Read the model definition and answer for the solid it produces. Units are mm, in the model's axes. A direction names the side the tool comes from. Give positions to 0.01 mm unless a question says otherwise; leave off trailing zeros. Write each loop counter-clockwise with the first axis right and the second up, starting at its lowest first coordinate (ties: lowest second). Pieces come first, ordered by that corner, then holes. Notation, with made-up numbers: (33.25, 69) - (43.25, 69) arc R21 cw to (43.25, 102) - close; hole circle Ø6 at (47.25, 89). An arc over 180 degrees is marked (long way). Answer as CSV lines item,"result".
```python
from build123d import *

# Parameters (mm, degrees)
TUBE_R                   = 5
TUBE_R_2                 = 4
TUBE_DEPTH               = 24
TUBE_PLACEMENT_ANGLE     = 70
BOX002_W                 = 13
BOX002_H                 = 4
BOX002_DEPTH             = 16
BOX001_W                 = 15
BOX001_H                 = 5
BOX001_DEPTH             = 18
CYLINDER_R               = 4
CYLINDER_DEPTH           = 35
CYLINDER_PLACEMENT_ANGLE = 70
BOX_W                    = 50
BOX_H                    = 100
BOX_DEPTH                = 2.6
EXTRUDE_DEPTH            = 10
EXTRUDE_PLACEMENT_ANGLE  = 70


with BuildPart() as tube:
    # Tube → Tube (new body)
    with BuildSketch(Plane.XY):
        Circle(TUBE_R)
        Circle(TUBE_R_2, mode=Mode.SUBTRACT)
    extrude(amount=TUBE_DEPTH)


with BuildPart() as tube_1:
    # Tube placement: moved
    add(tube.part.moved(Location((25.1, 89, -0.7))).rotate(Axis((25.1, 89, -0.7), (1, 0, 0)), TUBE_PLACEMENT_ANGLE))


with BuildPart() as cube002:
    # Box002 → Box002 (new body)
    with BuildSketch(Plane(origin=(18.5, 45, -6), x_dir=(1, 0, 0), z_dir=(0, 0, 1))):
        with Locations((6.5, 2)):
            Rectangle(BOX002_W, BOX002_H)
    extrude(amount=BOX002_DEPTH)


with BuildPart() as cut001:
    # Box001 → Box001 (new body)
    with BuildSketch(Plane(origin=(17.5, 45, -7.13), x_dir=(1, 0, 0), z_dir=(0, 0, 1))):
        with Locations((7.5, 2.5)):
            Rectangle(BOX001_W, BOX001_H)
    extrude(amount=BOX001_DEPTH)

    # Cut001: cut Cube002
    add(cube002.part, mode=Mode.SUBTRACT)


with BuildPart() as cut001_1:
    # Cut001 placement: moved
    add(cut001.part.moved(Location((0, 50, -8.5))))


with BuildPart() as cylinder:
    # Cylinder → Cylinder (new body)
    with BuildSketch(Plane.XY):
        Circle(CYLINDER_R)
    extrude(amount=CYLINDER_DEPTH)


with BuildPart() as cylinder_1:
    # Cylinder placement: moved
    add(cylinder.part.moved(Location((25.1, 98, -4))).rotate(Axis((25.1, 98, -4), (1, 0, 0)), CYLINDER_PLACEMENT_ANGLE))


with BuildPart() as cut:
    # Box → Box (new body)
    with BuildSketch(Plane.XY):
        with Locations((25, 50)):
            Rectangle(BOX_W, BOX_H)
    extrude(amount=BOX_DEPTH)

    # Cut: cut Cylinder
    add(cylinder_1.part, mode=Mode.SUBTRACT)


with BuildPart() as fusion:
    # Sketch → Extrude (new body)
    with BuildSketch(Plane.XY):
        with BuildLine():
            ThreePointArc((29.005047, 25.145956), (25.102383, 29.048619), (21.199722, 25.145954))
            Line((21.199722, 25.145954), (20.095131, 25.124403))
            ThreePointArc((30.109684, 25.145956), (25.091608, 30.153244), (20.095131, 25.124403))
            Line((29.005047, 25.145956), (30.109684, 25.145956))
        make_face()
    extrude(amount=EXTRUDE_DEPTH)


with BuildPart() as fusion_1:
    # Extrude placement: moved
    add(fusion.part.moved(Location((0, 89.5, -27.7))).rotate(Axis((0, 89.5, -27.7), (1, 0, 0)), EXTRUDE_PLACEMENT_ANGLE))

    # Fusion: union Tube, Cut001, Cut
    add(tube_1.part)
    add(cut001_1.part)
    add(cut.part)


solid = fusion_1.part
```
(1) Find the intervals of material crossed by L1, parallel to X at y = 82, z = 1.5; L2, parallel to Z at x = 47, y = 28; L3, parallel to Y at x = 27.5, z = -8.25, in increasing order.
Worked out:
L1,"x = 0 to 21.11, 29.09 to 50"
L2,"z = 0 to 2.6"
L3,"y = 99 to 100"
(2) A cutting plane is placed at C-C (y = 38). Write down the section's boundary in (x, z).
Worked out:
outline,"(0, 0) - (50, 0) - (50, 2.6) - (0, 2.6) - close"
(3) A cutting plane is placed at B-B (x = 39.5). Write down the section's boundary in (y, z), and give its area (3 significant figures).
Worked out:
outline,"(0, 0) - (100, 0) - (100, 2.6) - (0, 2.6) - close"
area,"260 mm^2"
(4) For faces 1 (the flat face through (18.5, 97, -7)), 2 (the flat face through (25, 0, 1)), 3 (the flat face through (32.5, 97, -8)), 4 (the cylindrical face through (20.456, 95.15, -1.012)), determine the directions among +Z, -Z, +X, -X, +Y, -Y from which every point of the face is accessible in a straight line to the end or side of a thin tool.
Worked out:
face 1,"-Y"
face 2,"+Z, -Z, +X, -X, -Y"
face 3,"-Z, +X, +Y, -Y"
face 4,"none"
(5) A cutting plane is placed at A-A (z = -6.75). Write down the section's boundary in (x, y), and give its area (3 significant figures).
Worked out:
outline,"(17.5, 95) - (18.5, 95) - (18.5, 99) - (31.5, 99) - (31.5, 95) - (32.5, 95) - (32.5, 100) - (17.5, 100) - close"
area,"23.0 mm^2"
(6) Each of these flat-tipped pins is pushed along its axis until it touches: P1, Ø10, axis at x = 39.5, y = 17.5, coming from the -Z side; P2, Ø0.6, axis at x = 22.5, y = 86, coming from the +Z side; P3, Ø1.2, axis at y = 97.5, z = -11, coming from the -X side; P4, Ø12, axis at x = 28.5, y = 67, coming from the +Z side. Where does it stop, or does it pass through?
Worked out:
P1,"stops at z = 0"
P2,"stops at z = 5.15"
P3,"stops at x = 17.5"
P4,"stops at z = 12.21"
(7) The mould has two halves that part along Y. Classify faces 5 (the flat face through (50, 49, 1)), 6 (the flat face through (24, 95, -15)), 7 (the flat face through (29.55, 93.468, -2.384)): +Y half, -Y half, draft (parallel to the pull), parting line (faces both ways), or undercut.
Worked out:
face 5,"draft"
face 6,"-Y half"
face 7,"undercut"
